For this review, take the finished solid that the model builds, in its own axes (mm). A direction names the side the tool comes from. Give positions to 0.01 mm unless a question says otherwise; leave off trailing zeros. Order: outer loops, then holes, each group sorted by start corner. A loop starts at its lowest first (then second) coordinate and runs counter-clockwise, first axis right, second up. Notation, with made-up numbers: (-11.75, 63) - (32.25, 63) arc R22 ccw to (32.25, 79) - close; hole circle Ø7 at (82.5, 55). An arc over 180 degrees is marked (long way). One line per item, written item: value.
Solid Edge part; units mm, degrees
sketch "Sketch1" plane through (0, 0, 0) normal (0, 0, 1) x (1, 0, 0)
  circle A0 centre (-98.8815, 36.1965) radius 500
extrude "Protrusion1" add sketch "Sketch1" along normal blind 10
sketch "Sketch2" plane through (-98.8815, 36.1965, 0) normal (0, 0, -1) x (1, 0, 0)
  circle A0 centre (0, 0) radius 100
extrude "ExtrudedProtrusion_2" add sketch "Sketch2" along normal blind 50
sketch "Sketch3" plane through (-98.8815, 36.1965, 10) normal (0, 0, 1) x (1, 0, 0)
  line L0 (-250, 350) -> (-250, -350)
  line L1 (-250, -350) -> (250, -350)
  line L2 (250, -350) -> (250, 350)
  line L3 (250, 350) -> (-250, 350)
  dimension "D1" = 250
  dimension "D2" = 250
extrude "ExtrudedProtrusion_3" add sketch "Sketch3" along normal blind 1
properties material "Aluminum, 6061-T6"
(1) Take a section at A-A (x = 102.5). Write out the cut boundary in (y, z), then the cut area to 3 significant figures.
Answers below:
outline: (-421.46, 0) - (493.85, 0) - (493.85, 10) - (386.2, 10) - (386.2, 11) - (-313.8, 11) - (-313.8, 10) - (-421.46, 10) - close
area: 9,850 mm^2
(2) Machinability: for faces 1 (the face through (378.03, -113.99, 4.93)), 2 (the face through (-111.9, 135.346, -24.65)), which of the approach directions +Z, -Z, +X, -X, +Y, -Y give a long, thin tool a straight path to every point of the face, cutting with its end or side? Answer none if there is none.
Answers below:
face 1: +Z, -Z
face 2: -Z
(3) Wall thickness on line 1 (Z direction, x = 297, y = 257); line 2 (Z direction, x = 56.5, y = -181); line 3 (Y direction, x = -251.5, z = 7.5): over which ranges is each line inside the solid? List them lowest first. Write a range as from..to.
Answers below:
line 1: z = 0..10
line 2: z = 0..11
line 3: y = -439.94..512.33
(4) Take a section at C-C (x = -130). Write out the cut boundary in (y, z).
Answers below:
outline: (-462.83, 0) - (-58.84, 0) - (-58.84, -50) - (131.23, -50) - (131.23, 0) - (535.23, 0) - (535.23, 10) - (386.2, 10) - (386.2, 11) - (-313.8, 11) - (-313.8, 10) - (-462.83, 10) - close
(5) For P1, Ø4, axis at x = -201, z = 0, coming from the -Y side; P2, Ø8, axis at y = 404, z = 4, coming from the -X side; P3, Ø6, axis at x = 207.5, y = 83.5, coming from the +Z side, all flat-tipped, find the tip position at first contact; note any pin that passes through.
Answers below:
P1: stops at y = -453.68
P2: stops at x = -441.88
P3: stops at z = 10
(6) Take a section at D-D (y = -12.5). Write out the cut boundary in (x, z).
Answers below:
outline: (-596.5, 0) - (-186.22, 0) - (-186.22, -50) - (-11.54, -50) - (-11.54, 0) - (398.74, 0) - (398.74, 10) - (151.12, 10) - (151.12, 11) - (-348.88, 11) - (-348.88, 10) - (-596.5, 10) - close
(7) Take a section at B-B (y = -270.5). Write out the cut boundary in (x, z).
Answers below:
outline: (-493.77, 0) - (296.01, 0) - (296.01, 10) - (151.12, 10) - (151.12, 11) - (-348.88, 11) - (-348.88, 10) - (-493.77, 10) - close
